from build123d import *

# Parameters (mm, degrees)
SKETCH1_W            = 100
SKETCH1_H            = 140
BOSS_EXTRUDE1_DEPTH  = 3
BOSS_EXTRUDE2_DEPTH  = 22.3
SKETCH4_W            = 3.5
SKETCH4_H            = 5.5
CUT_EXTRUDE2_DEPTH   = 5
CUT_EXTRUDE1_START   = -3
SKETCH3_R            = 1.5
CUT_EXTRUDE1_DEPTH   = 22.7
BOSS_EXTRUDE3_DEPTH  = 18
BOSS_EXTRUDE4_DEPTH  = 3
SKETCH7_W            = 26
SKETCH7_H            = 18
BOSS_EXTRUDE5_DEPTH  = 6
BOSS_EXTRUDE8_DEPTH  = 3
SKETCH9_R            = 2.6
SKETCH9_R_2          = 1.6
BOSS_EXTRUDE7_DEPTH  = 4
BOSS_EXTRUDE9_DEPTH  = 18
SKETCH13_R           = 1.6
BOSS_EXTRUDE10_DEPTH = 18
CUT_EXTRUDE3_REACH   = 5
SKETCH12_R           = 4.1
SKETCH14_R           = 0.75
CUT_EXTRUDE4_DEPTH   = 2
CUT_EXTRUDE5_DEPTH   = 2
FILLET2_R            = 8


with BuildPart() as part:
    # Sketch1 → Boss-Extrude1 (new body)
    with BuildSketch(Plane(origin=(0, 0, 0), x_dir=(1, 0, 0), z_dir=(0, 1, 0))):
        Rectangle(SKETCH1_W, SKETCH1_H)
    extrude(amount=BOSS_EXTRUDE1_DEPTH)

    # Sketch2 → Boss-Extrude2 (add)
    with BuildSketch(Plane(origin=(0, 3, 0), x_dir=(1, 0, 0), z_dir=(0, 1, 0))):
        Polygon((-50, -65), (-50, -70), (-28.3, -70), (-28.3, -28), (-31.3, -28), (-31.3, -65), align=None)
    boss_extrude2 = extrude(amount=BOSS_EXTRUDE2_DEPTH)

    # Sketch4 → Cut-Extrude2 (cut)
    with BuildSketch(Plane(origin=(0, 0, 65), x_dir=(-1, 0, 0), z_dir=(0, 0, -1))):
        with Locations((40.3, 14.15)):
            Rectangle(SKETCH4_W, SKETCH4_H)
    cut_extrude2 = extrude(amount=-CUT_EXTRUDE2_DEPTH, mode=Mode.SUBTRACT)

    # Sketch3 → Cut-Extrude1 (cut)
    with BuildSketch(Plane.ZY.offset(31.3).offset(CUT_EXTRUDE1_START)):
        with Locations((67, 14.15)):
            Circle(SKETCH3_R)
        with BuildLine():
            Line((53.5, 10.65), (48.5, 10.65))
            ThreePointArc((48.5, 10.65), (45, 14.15), (48.5, 17.65))
            Line((48.5, 17.65), (53.5, 17.65))
            ThreePointArc((53.5, 17.65), (57, 14.15), (53.5, 10.65))
        make_face()
    cut_extrude1 = extrude(amount=CUT_EXTRUDE1_DEPTH, mode=Mode.SUBTRACT)

    # Mirror1: Boss-Extrude2, Cut-Extrude2, Cut-Extrude1 across plane
    add(boss_extrude2.mirror(Plane(origin=(0, 0, 0), x_dir=(0, 0, 1), z_dir=(1, 0, 0))))
    add(cut_extrude2.mirror(Plane(origin=(0, 0, 0), x_dir=(0, 0, 1), z_dir=(1, 0, 0))), mode=Mode.SUBTRACT)
    add(cut_extrude1.mirror(Plane(origin=(0, 0, 0), x_dir=(0, 0, 1), z_dir=(1, 0, 0))), mode=Mode.SUBTRACT)

    # Sketch5 → Boss-Extrude3 (add)
    with BuildSketch(Plane(origin=(0, 3, 0), x_dir=(1, 0, 0), z_dir=(0, 1, 0))):
        Polygon((13, -70), (16, -70), (16, 3), (-16, 3), (-16, -70), (-13, -70), (-13, 0), (13, 0), align=None)
    extrude(amount=BOSS_EXTRUDE3_DEPTH)

    # Sketch6 → Boss-Extrude4 (add)
    with BuildSketch(Plane.XY.offset(70)):
        Polygon((28.3, 25.3), (28.3, 3), (16, 3), (16, 21), (13, 21), (-13, 21), (-16, 21), (-16, 3), (-28.3, 3), (-28.3, 25.3), align=None)
    extrude(amount=-BOSS_EXTRUDE4_DEPTH)

    # Sketch7 → Boss-Extrude5 (add)
    with BuildSketch(Plane.XY.offset(70)):
        with BuildLine():
            Line((-12, 23), (12, 23))
            ThreePointArc((12, 23), (14.121320344, 22.121320344), (15, 20))
            Line((15, 20), (15, 4))
            ThreePointArc((15, 4), (14.121320344, 1.878679656), (12, 1))
            Line((12, 1), (-12, 1))
            ThreePointArc((-12, 1), (-14.121320344, 1.878679656), (-15, 4))
            Line((-15, 4), (-15, 20))
            ThreePointArc((-15, 20), (-14.121320344, 22.121320344), (-12, 23))
        make_face()
        with Locations((0, 12)):
            Rectangle(SKETCH7_W, SKETCH7_H, mode=Mode.SUBTRACT)
    extrude(amount=BOSS_EXTRUDE5_DEPTH)

    # Sketch10 → Boss-Extrude8 (add)
    with BuildSketch(Plane(origin=(0, 3, 0), x_dir=(1, 0, 0), z_dir=(0, 1, 0))):
        Polygon((50, 70), (-50, 70), (0, 130), align=None)
    extrude(amount=-BOSS_EXTRUDE8_DEPTH)

    # Sketch9 → Boss-Extrude7 (add)
    with BuildSketch(Plane(origin=(0, 3, 0), x_dir=(1, 0, 0), z_dir=(0, 1, 0))):
        with Locations((-34.7, 54.2)):
            Circle(SKETCH9_R)
        with Locations((-34.7, 54.2)):
            Circle(SKETCH9_R_2, mode=Mode.SUBTRACT)
        with Locations((-36, 6)):
            Circle(SKETCH9_R)
        with Locations((-36, 6)):
            Circle(SKETCH9_R_2, mode=Mode.SUBTRACT)
        with Locations((16.1, 10.8)):
            Circle(SKETCH9_R)
        with Locations((16.1, 10.8)):
            Circle(SKETCH9_R_2, mode=Mode.SUBTRACT)
        with Locations((16.1, 38.7)):
            Circle(SKETCH9_R)
        with Locations((16.1, 38.7)):
            Circle(SKETCH9_R_2, mode=Mode.SUBTRACT)
        with Locations((-18.5, 62.2)):
            Circle(SKETCH9_R)
        with Locations((-18.5, 62.2)):
            Circle(SKETCH9_R_2, mode=Mode.SUBTRACT)
        with Locations((-18.5, 99.2)):
            Circle(SKETCH9_R)
        with Locations((-18.5, 99.2)):
            Circle(SKETCH9_R_2, mode=Mode.SUBTRACT)
        with Locations((18.5, 99.2)):
            Circle(SKETCH9_R)
        with Locations((18.5, 99.2)):
            Circle(SKETCH9_R_2, mode=Mode.SUBTRACT)
        with Locations((18.5, 62.2)):
            Circle(SKETCH9_R)
        with Locations((18.5, 62.2)):
            Circle(SKETCH9_R_2, mode=Mode.SUBTRACT)
    extrude(amount=BOSS_EXTRUDE7_DEPTH)

    # Sketch11 → Boss-Extrude9 (add)
    with BuildSketch(Plane(origin=(0, 3, 0), x_dir=(1, 0, 0), z_dir=(0, 1, 0))):
        Polygon((50, 5), (50, 70), (35, 88), (27, 88), (27, 97.6), (25, 100), (25, 96.87590013), (25, 86), (27, 86), (34.063250108, 86), (48, 69.27590013), (48, 62), (27, 62), (27, 68), (25, 68), (25, 60), (48, 60), (48, 7), (22, 7), (22, 52), (20, 52), (20, 5), align=None)
        Polygon((-50, 70), (-50, 60), (-25, 60), (-25, 68), (-27, 68), (-27, 62), (-48, 62), (-48, 69.27590013), (-34.063250108, 86), (-27, 86), (-25, 86), (-25, 96.87590013), (-25, 100), (-27, 97.6), (-27, 88), (-35, 88), align=None)
    extrude(amount=BOSS_EXTRUDE9_DEPTH)

    # Sketch13 → Boss-Extrude10 (add)
    with BuildSketch(Plane(origin=(0, 3, 0), x_dir=(1, 0, 0), z_dir=(0, 1, 0))):
        with BuildLine():
            Line((16, 2.368543856), (16, 3))
            Line((16, 3), (17.218975032, 3))
            ThreePointArc((17.218975032, 3), (19.425906443, -2.752597104), (16, 2.368543856))
        make_face()
        with Locations((18, 0)):
            Circle(SKETCH13_R, mode=Mode.SUBTRACT)
        with BuildLine():
            Line((27, 66.368543856), (27, 68))
            Line((27, 68), (30.037478421, 66.921239211))
            ThreePointArc((30.037478421, 66.921239211), (29.554959445, 60.950078687), (27, 66.368543856))
        make_face()
        with Locations((29, 64)):
            Circle(SKETCH13_R, mode=Mode.SUBTRACT)
    boss_extrude10 = extrude(amount=BOSS_EXTRUDE10_DEPTH)

    # Sketch12 → Cut-Extrude3 (cut, up to next)
    with BuildSketch(Plane(origin=(0, 3, 0), x_dir=(1, 0, 0), z_dir=(0, 1, 0)), mode=Mode.PRIVATE) as cut_extrude3_sk1:
        with Locations((0, 114.379500648)):
            Circle(SKETCH12_R)
    cut_extrude3_tool1 = extrude(cut_extrude3_sk1.sketch, amount=-CUT_EXTRUDE3_REACH, mode=Mode.PRIVATE) & part.part
    add(cut_extrude3_tool1.solids().sort_by_distance((0, 3, -114.379501))[0], mode=Mode.SUBTRACT)
    # Sketch12 → Cut-Extrude3 (cut, up to next)
    with BuildSketch(Plane(origin=(0, 3, 0), x_dir=(1, 0, 0), z_dir=(0, 1, 0)), mode=Mode.PRIVATE) as cut_extrude3_sk2:
        with BuildLine():
            Line((7.682212796, 120.781344645), (0, 130))
            Line((0, 130), (-7.682212796, 120.781344645))
            ThreePointArc((-7.682212796, 120.781344645), (0, 124.379500648), (7.682212796, 120.781344645))
        make_face()
    cut_extrude3_tool2 = extrude(cut_extrude3_sk2.sketch, amount=-CUT_EXTRUDE3_REACH, mode=Mode.PRIVATE) & part.part
    add(cut_extrude3_tool2.solids().sort_by_distance((0, 3, -125.762596))[0], mode=Mode.SUBTRACT)

    # Sketch14 → Cut-Extrude4 (cut)
    with BuildSketch(Plane(origin=(0, 0, -88), x_dir=(-1, 0, 0), z_dir=(0, 0, -1))):
        with Locations((-29, 12)):
            Circle(SKETCH14_R)
        with Locations((-33, 12)):
            Circle(SKETCH14_R)
    cut_extrude4 = extrude(amount=-CUT_EXTRUDE4_DEPTH, mode=Mode.SUBTRACT)

    # Sketch15 → Cut-Extrude5 (cut)
    with BuildSketch(Plane(origin=(0, 0, -62), x_dir=(-1, 0, 0), z_dir=(0, 0, -1))):
        with BuildLine():
            Line((-44.684271928, 21), (-34.684271928, 21))
            ThreePointArc((-34.684271928, 21), (-39.684271928, 16), (-44.684271928, 21))
        make_face()
    cut_extrude5 = extrude(amount=-CUT_EXTRUDE5_DEPTH, mode=Mode.SUBTRACT)

    # Fillet2
    fillet2_edges = [part.edges().sort_by_distance(p)[0] for p in [
        (48, 12, -69.27590013),
        (-48, 12, -69.27590013),
        (-50, 10.5, -70),
        (50, 10.5, -70),
    ]]
    fillet(fillet2_edges, radius=FILLET2_R)

    # Mirror2: Boss-Extrude10, Cut-Extrude4, Cut-Extrude5 across plane
    add(boss_extrude10.mirror(Plane(origin=(0, 0, 0), x_dir=(0, 0, 1), z_dir=(1, 0, 0))))
    add(cut_extrude4.mirror(Plane(origin=(0, 0, 0), x_dir=(0, 0, 1), z_dir=(1, 0, 0))), mode=Mode.SUBTRACT)
    add(cut_extrude5.mirror(Plane(origin=(0, 0, 0), x_dir=(0, 0, 1), z_dir=(1, 0, 0))), mode=Mode.SUBTRACT)


solid = part.part
Could you check a few things on this model? Use its own coordinates, in mm. A direction names the side the tool comes from. Give positions to 0.01 mm unless a question says otherwise; leave off trailing zeros. Order: outer loops, then holes, each group sorted by start corner. A loop starts at its lowest first (then second) coordinate and runs counter-clockwise, first axis right, second up. Notation, with made-up numbers: (22.5, 34) - (66.5, 34) arc R23 cw to (66.5, 53) - close; hole circle Ø10 at (-7, 30). An arc over 180 degrees is marked (long way). Return JSON: item names as keys, results as strings. Group by question number.
Q1. Which directions (+Z, -Z, +X, -X, +Y, -Y) give clear straight access to the entire face, cutting with the end or side of a thin tool? Please do faces 4 (the face through (-25, 12, -64)), 5 (the face through (0, 1, 73)), 6 (the face through (-29, 3, -91)), 7 (the face through (-38.55, 14, 69)).
Q2. Suppose I cut it at A-A, the plane z = 63. Please give me the cut outline in (x, y), and give its area (3 significant figures).
Q3. Suppose I cut it at B-B, the plane z = 23. Please give me the cut outline in (x, y).
Q4. Will these pins go through, and if not, where does the flat tip stop? pin 1 Ø1.6 at (x, z) = (-18.5, 0.5) entering from +Y; pin 2 Ø6.5 at (x, z) = (1.5, 73.5) entering from -Y; pin 3 Ø12 at (x, z) = (-35.5, 4.5) entering from -Y; pin 4 Ø10 at (y, z) = (14.5, 36) entering from +X.
Q5. Please list where these lines run through material, in increasing order: line 1 along X through (y, z) = (15.75, 39); line 2 along Z through (x, y) = (33.25, 14.15); line 3 along Y through (x, z) = (-48.25, 67). Write a range as [from, to].
Q6. Thinking about a two-plate mould opening in Z: for faces 1 (the face through (37.19, 8.02, -85.37)), 2 (the face through (31.98, 11.87, -64.85)), 3 (the face through (-50, 1, 1)), which applies, pulls with the +Z half, pulls with the -Z half, needs draft (parallel to the pull), parting line crosses it, or undercut?
Resolved:
{
 "1": {"face 4": "-Z, +Y", "face 5": "+Z, +X, -X, -Y", "face 6": "-Z, -X, +Y", "face 7": "+Z"},
 "2": {"outline": "(-50, 0) - (50, 0) - (50, 3) - (31.3, 3) - (31.3, 25.3) - (28.3, 25.3) - (28.3, 3) - (16, 3) - (16, 21) - (13, 21) - (13, 3) - (-13, 3) - (-13, 21) - (-16, 21) - (-16, 3) - (-28.3, 3) - (-28.3, 25.3) - (-31.3, 25.3) - (-31.3, 3) - (-50, 3) - close", "area": "542 mm2"},
 "3": {"outline": "(-50, 0) - (50, 0) - (50, 3) - (16, 3) - (16, 21) - (13, 21) - (13, 3) - (-13, 3) - (-13, 21) - (-16, 21) - (-16, 3) - (-50, 3) - close"},
 "4": {"pin 1": "stops at y = 3", "pin 2": "stops at y = 1", "pin 3": "stops at y = 0", "pin 4": "stops at x = 31.3"},
 "5": {"line 1": "x = [-31.3, -28.3], [-16, -13], [13, 16], [28.3, 31.3]", "line 2": "z = [-88, -86], [-62, -60], [-7, -5], [65, 65.5], [68.5, 70]", "line 3": "y = [0, 12.65], [15.65, 25.3]"},
 "6": {"face 1": "pulls with the -Z half", "face 2": "undercut", "face 3": "needs draft"}
}
